Could you check a few things on this model? Use its own coordinates, in mm. Coordinates: 2 decimals unless noted, no trailing zeros. Answer as CSV lines item,"result". Start each with the question number.
Item 1: I'm going to push flat-ended pins straight in: P1, Ø4.5, axis at x = 38.1, z = -319.09, coming from the +Y side; P2, Ø10, axis at x = 41.5, z = -36, coming from the -Y side. Where does each tip first touch, or does it pass through?
Item 2: Suppose I cut it at A-A, the plane y = 0.35. State how many separate pieces and enclosed holes the cut face has, and give its area (3 significant figures).
Item 3: If I drill on line 1 along X through (y, z) = (1.45, -13.5); line 2 along Z through (x, y) = (48, 1.1), over which ranges is the centre line in solid material (lowest first)? Write a range as [from, to].
```python
from build123d import *

# Parameters (mm, degrees)
SKETCH1_W           = 50.8
SKETCH1_H           = 331.7875
SKETCH1_R           = 2.4892
BOSS_EXTRUDE1_DEPTH = 1.5875
FILLET1_R           = 3.175


with BuildPart() as part:
    # Sketch1 → Boss-Extrude1 (new body)
    with BuildSketch(Plane(origin=(0, 0, 0), x_dir=(1, 0, 0), z_dir=(0, 1, 0))):
        with Locations((25.4, 165.89375)):
            Rectangle(SKETCH1_W, SKETCH1_H)
        with Locations(Location((12.7, 14.2875, 0), (0, 0, 270))):
            Circle(SKETCH1_R, mode=Mode.SUBTRACT)
        with Locations(Location((12.7, 39.6875, 0), (0, 0, 270))):
            Circle(SKETCH1_R, mode=Mode.SUBTRACT)
        with Locations(Location((12.7, 65.0875, 0), (0, 0, 270))):
            Circle(SKETCH1_R, mode=Mode.SUBTRACT)
        with Locations(Location((12.7, 90.4875, 0), (0, 0, 270))):
            Circle(SKETCH1_R, mode=Mode.SUBTRACT)
        with Locations(Location((12.7, 115.8875, 0), (0, 0, 270))):
            Circle(SKETCH1_R, mode=Mode.SUBTRACT)
        with Locations(Location((12.7, 141.2875, 0), (0, 0, 270))):
            Circle(SKETCH1_R, mode=Mode.SUBTRACT)
        with Locations(Location((38.1, 39.6875, 0), (0, 0, 270))):
            Circle(SKETCH1_R, mode=Mode.SUBTRACT)
        with Locations(Location((38.1, 65.0875, 0), (0, 0, 270))):
            Circle(SKETCH1_R, mode=Mode.SUBTRACT)
        with Locations(Location((38.1, 90.4875, 0), (0, 0, 270))):
            Circle(SKETCH1_R, mode=Mode.SUBTRACT)
        with Locations(Location((38.1, 115.8875, 0), (0, 0, 270))):
            Circle(SKETCH1_R, mode=Mode.SUBTRACT)
        with Locations(Location((38.1, 141.2875, 0), (0, 0, 270))):
            Circle(SKETCH1_R, mode=Mode.SUBTRACT)
        with Locations(Location((38.1, 14.2875, 0), (0, 0, 270))):
            Circle(SKETCH1_R, mode=Mode.SUBTRACT)
        with Locations(Location((12.7, 166.6875, 0), (0, 0, 270))):
            Circle(SKETCH1_R, mode=Mode.SUBTRACT)
        with Locations(Location((38.1, 166.6875, 0), (0, 0, 270))):
            Circle(SKETCH1_R, mode=Mode.SUBTRACT)
        with Locations(Location((12.7, 319.0875, 0), (0, 0, 270))):
            Circle(SKETCH1_R, mode=Mode.SUBTRACT)
        with Locations(Location((38.1, 319.0875, 0), (0, 0, 270))):
            Circle(SKETCH1_R, mode=Mode.SUBTRACT)
        with Locations(Location((12.7, 293.6875, 0), (0, 0, 270))):
            Circle(SKETCH1_R, mode=Mode.SUBTRACT)
        with Locations(Location((38.1, 293.6875, 0), (0, 0, 270))):
            Circle(SKETCH1_R, mode=Mode.SUBTRACT)
        with Locations(Location((12.7, 268.2875, 0), (0, 0, 270))):
            Circle(SKETCH1_R, mode=Mode.SUBTRACT)
        with Locations(Location((38.1, 268.2875, 0), (0, 0, 270))):
            Circle(SKETCH1_R, mode=Mode.SUBTRACT)
        with Locations(Location((12.7, 242.8875, 0), (0, 0, 270))):
            Circle(SKETCH1_R, mode=Mode.SUBTRACT)
        with Locations(Location((38.1, 242.8875, 0), (0, 0, 270))):
            Circle(SKETCH1_R, mode=Mode.SUBTRACT)
        with Locations(Location((12.7, 217.4875, 0), (0, 0, 270))):
            Circle(SKETCH1_R, mode=Mode.SUBTRACT)
        with Locations(Location((38.1, 217.4875, 0), (0, 0, 270))):
            Circle(SKETCH1_R, mode=Mode.SUBTRACT)
        with Locations(Location((12.7, 192.0875, 0), (0, 0, 270))):
            Circle(SKETCH1_R, mode=Mode.SUBTRACT)
        with Locations(Location((38.1, 192.0875, 0), (0, 0, 270))):
            Circle(SKETCH1_R, mode=Mode.SUBTRACT)
    extrude(amount=BOSS_EXTRUDE1_DEPTH)

    # Fillet1
    fillet1_edges = [part.edges().sort_by_distance(p)[0] for p in [
        (0, 0.79375, -331.7875),
        (50.8, 0.79375, -331.7875),
        (50.8, 0.79375, 0),
        (0, 0.79375, 0),
    ]]
    fillet(fillet1_edges, radius=FILLET1_R)


solid = part.part
```
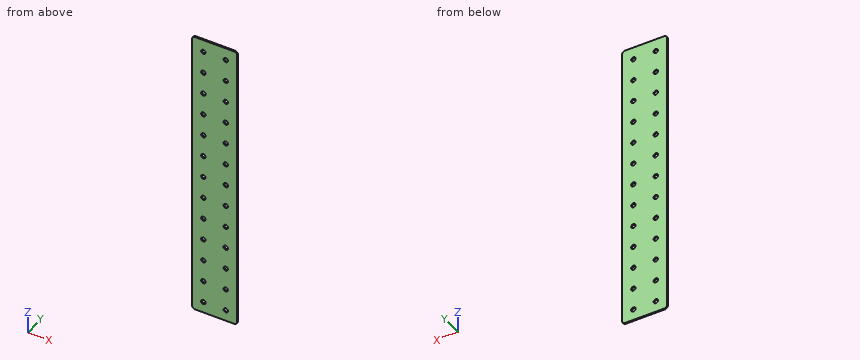
Ans:
1,P1,"passes through"
1,P2,"stops at y = 0"
2,separate pieces,"1"
2,enclosed holes,"26"
2,area,"16,300 mm^2"
3,line 1,"x = [0, 10.34], [15.06, 35.74], [40.46, 50.8]"
3,line 2,"z = [-331.77, -0.02]"
